```python
from build123d import *

# Parameters (mm, degrees)
SKETCH_1_W          = 60
SKETCH_1_H          = 59
EXTRUDE_1_DEPTH     = 8
SKETCH_2_R          = 1.25
CUT_EXTRUDE_1_DEPTH = 8
SKETCH_3_R          = 1.6
CUT_EXTRUDE_2_DEPTH = 85.528101836


with BuildPart() as part:
    # 草图1 → 凸台-拉伸1 (new body)
    with BuildSketch(Plane.XY):
        with Locations((30, -29.5)):
            Rectangle(SKETCH_1_W, SKETCH_1_H)
    extrude(amount=EXTRUDE_1_DEPTH)

    # 草图2 → 切除-拉伸1 (cut)
    with BuildSketch(Plane.XY.offset(8)):
        with Locations((11.5, -4.5)):
            Circle(SKETCH_2_R)
        with Locations((48.5, -4.5)):
            Circle(SKETCH_2_R)
        with Locations((11.5, -41.5)):
            Circle(SKETCH_2_R)
        with Locations((48.5, -41.5)):
            Circle(SKETCH_2_R)
    extrude(amount=-CUT_EXTRUDE_1_DEPTH, mode=Mode.SUBTRACT)

    # 草图3 → 切除-拉伸2 (cut, through all)
    with BuildSketch(Plane.XY.offset(8)):
        with Locations((10, -55)):
            Circle(SKETCH_3_R)
        with Locations((20, -55)):
            Circle(SKETCH_3_R)
        with Locations((30, -55)):
            Circle(SKETCH_3_R)
        with Locations((40, -55)):
            Circle(SKETCH_3_R)
        with Locations((50, -55)):
            Circle(SKETCH_3_R)
    extrude(amount=-CUT_EXTRUDE_2_DEPTH, mode=Mode.SUBTRACT)


solid = part.part
```
Geometry check sheet. Reference: the model listing, model coordinates, mm. Give positions to 0.01 mm unless a question says otherwise; leave off trailing zeros. Loops run counter-clockwise (first coordinate to the right, second up) from the corner with the lowest first, then second, coordinate; pieces in that order, holes last. Notation, with made-up numbers: M -12.75,-11.5 L -6.75,-11.5 A5 cw -6.75,-7.5 Z; hole C -7.5,2.5 d5. An arc over 180 degrees is marked long. Write item = value, one per line. Start each with the question number.
1. Section check C-C, the plane y = -55. Enter the section's corners in (x, z), plus the area to 3 significant figures.
2. Draft check along X on faces 1 (the face through (0, -30, 4)), 2 (the face through (30, -29, 0)), 3 (the face through (8.4, -54.93, 4.06)). Enter one of: +X half, -X half, draft (parallel to the pull), parting line (faces both ways), or undercut.
3. Section check B-B, the plane y = -41.5. Enter the section's corners in (x, z).
4. Go/stop test with a flat-tipped pin: P1, Ø2.5, axis at x = 40, y = -55, coming from the -Z side (3 decimals). Record where the tip stops, or that it passes through.
5. Section check A-A, the plane x = 20. Enter the section's corners in (y, z).
6. Thickness scan on probe 1 along Y at (x, z) = (30, 5). Record the ranges inside material, lowest first.
7. Section check D-D, the plane z = 3. Give the number of separate pieces and of enclosed holes in the cut face, plus the area to 3 significant figures.
Values follow:
q1.outline = M 0,0 L 8.4,0 L 8.4,8 L 0,8 Z; M 11.6,0 L 18.4,0 L 18.4,8 L 11.6,8 Z; M 21.6,0 L 28.4,0 L 28.4,8 L 21.6,8 Z; M 31.6,0 L 38.4,0 L 38.4,8 L 31.6,8 Z; M 41.6,0 L 48.4,0 L 48.4,8 L 41.6,8 Z; M 51.6,0 L 60,0 L 60,8 L 51.6,8 Z
q1.area = 352 mm^2
q2.face_1 = -X half
q2.face_2 = draft
q2.face_3 = undercut
q3.outline = M 0,0 L 10.25,0 L 10.25,8 L 0,8 Z; M 12.75,0 L 47.25,0 L 47.25,8 L 12.75,8 Z; M 49.75,0 L 60,0 L 60,8 L 49.75,8 Z
q4.P1 = through
q5.outline = M -59,0 L -56.6,0 L -56.6,8 L -59,8 Z; M -53.4,0 L 0,0 L 0,8 L -53.4,8 Z
q6.probe_1 = -59 to -56.6, -53.4 to 0
q7.separate_pieces = 1
q7.enclosed_holes = 9
q7.area = 3,480 mm^2
